The listing builds one solid part. Answer for the finished solid, in the listing's coordinates (mm). A direction names the side the tool comes from. Round coordinates to 2 decimals unless told otherwise and drop trailing zeros. Loops run counter-clockwise (first coordinate to the right, second up) from the corner with the lowest first, then second, coordinate; pieces in that order, holes last. Notation, with made-up numbers: (-14.5, 2) - (-6.5, 2) arc R19 cw to (-6.5, 35) - close; hole circle Ø1 at (11.25, -14). An arc over 180 degrees is marked (long way). One line per item, written item: value.
```python
from build123d import *

# Parameters (mm, degrees)
ESBO_O1_R                = 1.5
ESBO_O1_R_2              = 3.5
ESBO_O1_R_3              = 0.9
ESBO_O1_W                = 22.6
ESBO_O1_H                = 12.3
ESBO_O1_W_2              = 3
ESBO_O1_H_2              = 8
ESBO_O1_W_3              = 8
ESBO_O1_H_3              = 3
RESSALTO_EXTRUS_O1_DEPTH = 3


with BuildPart() as part:
    # Esboço1 → Ressalto-extrusão1 (new body)
    with BuildSketch(Plane(origin=(0, 0, 0), x_dir=(1, 0, 0), z_dir=(0, 1, 0))):
        with BuildLine():
            ThreePointArc((-26.75078073, 16.719697214), (-30.815641586, -2.3e-07), (-26.750780519, -16.719697622))
            ThreePointArc((-26.750780519, -16.719697622), (-23.767751269, -20.202130616), (-19.544028371, -21.987058612))
            add(Edge.make_bspline(
                [(23.247280819, -14.466941833), (22.21541658, -14.85491506), (7.843575487, -20.128766531), (-8.032505645, -23.945383183), (-19.544028371, -21.987058612)],
                knots=[0.1894974, 0.1894974, 0.1894974, 0.1894974, 0.216439611, 0.561126756, 0.561126756, 0.561126756, 0.561126756], degree=3))
            ThreePointArc((23.247280819, -14.466941833), (53.114593998, -6.632399806), (83.953283265, -5.079438247))
            add(Edge.make_bspline(
                [(97.598521861, -6.15), (93.039003458, -5.676054912), (88.490590593, -5.319200994), (83.953283265, -5.079438247)],
                knots=[0, 0, 0, 0, 0.137959586, 0.137959586, 0.137959586, 0.137959586], degree=3))
            add(Edge.make_bspline(
                [(114.569723425, -4.259468977), (109.134912936, -6.157348784), (103.477845748, -6.787525792), (97.598521861, -6.15)],
                knots=[0.35388944, 0.35388944, 0.35388944, 0.35388944, 1, 1, 1, 1], degree=3))
            ThreePointArc((114.569723425, -4.259468977), (117.037611185, -3.468795912), (119.543150354, -2.807050219))
            add(Edge.make_bspline(
                [(119.543150354, -2.807050219), (131.408766059, 0), (119.543150354, 2.807050219)],
                knots=[5.194112445, 5.194112445, 5.194112445, 7.372258169, 7.372258169, 7.372258169], degree=2, weights=[1, 0.463307193, 1]))
            ThreePointArc((119.543150354, 2.807050219), (117.037611185, 3.468795912), (114.569723425, 4.259468977))
            add(Edge.make_bspline(
                [(114.569723425, 4.259468977), (109.134912936, 6.157348784), (103.477845748, 6.787525792), (97.598521861, 6.15)],
                knots=[0.35388944, 0.35388944, 0.35388944, 0.35388944, 1, 1, 1, 1], degree=3))
            add(Edge.make_bspline(
                [(97.598521861, 6.15), (93.039003574, 5.676054924), (88.490590825, 5.319201013), (83.953283612, 5.079438265)],
                knots=[0, 0, 0, 0, 0.137959582, 0.137959582, 0.137959582, 0.137959582], degree=3))
            ThreePointArc((83.953283612, 5.079438265), (53.114594943, 6.632399691), (23.24728229, 14.466941345))
            add(Edge.make_bspline(
                [(23.24728229, 14.466941345), (22.21541757, 14.854914742), (7.843576153, 20.128766099), (-8.032505406, 23.945382333), (-19.544028008, 21.987058404)],
                knots=[0.189497388, 0.189497388, 0.189497388, 0.189497388, 0.216439611, 0.561126752, 0.561126752, 0.561126752, 0.561126752], degree=3))
            ThreePointArc((-19.544028008, 21.987058404), (-23.767751262, 20.202130438), (-26.75078073, 16.719697214))
        make_face()
        with Locations((-14.3, 0)):
            Circle(ESBO_O1_R, mode=Mode.SUBTRACT)
        with Locations((14.3, 0)):
            Circle(ESBO_O1_R, mode=Mode.SUBTRACT)
        with Locations((0.2, 14.3)):
            Circle(ESBO_O1_R, mode=Mode.SUBTRACT)
        with Locations((-22.8, -14.3)):
            Circle(ESBO_O1_R, mode=Mode.SUBTRACT)
        with Locations((-14.3, 11.5)):
            Circle(ESBO_O1_R, mode=Mode.SUBTRACT)
        with Locations((14.3, -11.5)):
            Circle(ESBO_O1_R, mode=Mode.SUBTRACT)
        with Locations((106.3, 0)):
            Circle(ESBO_O1_R_2, mode=Mode.SUBTRACT)
        with Locations((96.3, 0)):
            Circle(ESBO_O1_R_3, mode=Mode.SUBTRACT)
        with Locations((116.3, 0)):
            Circle(ESBO_O1_R_3, mode=Mode.SUBTRACT)
        with Locations((31.3, 0)):
            Circle(ESBO_O1_R, mode=Mode.SUBTRACT)
        with Locations((81.3, 0)):
            Circle(ESBO_O1_R, mode=Mode.SUBTRACT)
        Rectangle(ESBO_O1_W, ESBO_O1_H, mode=Mode.SUBTRACT)
        with Locations((0.2, -14.3)):
            Rectangle(ESBO_O1_W_2, ESBO_O1_H_2, mode=Mode.SUBTRACT)
        with Locations((-22.8, 14.3)):
            Rectangle(ESBO_O1_W_2, ESBO_O1_H_2, mode=Mode.SUBTRACT)
        with Locations((14.3, 11.500000009)):
            Rectangle(ESBO_O1_W_3, ESBO_O1_H_3, mode=Mode.SUBTRACT)
        with Locations((-14.3, -11.5)):
            Rectangle(ESBO_O1_W_3, ESBO_O1_H_3, mode=Mode.SUBTRACT)
        Polygon((56.3, -1.5), (60.3, -1.5), (60.3, 1.5), (52.3, 1.5), (52.3, -1.5), align=None, mode=Mode.SUBTRACT)
    extrude(amount=RESSALTO_EXTRUS_O1_DEPTH)


solid = part.part
```
1) For faces 1 (the cylindrical face through (117, 1.48, 3.48)), 2 (the flat face through (-14, 1, 10)), determine the directions among +Z, -Z, +X, -X, +Y, -Y from which every point of the face is accessible in a straight line to the end or side of a thin tool.
Final values:
face 1: +Z, +X, +Y, -Y
face 2: +Y, -Y
2) A cutting plane is placed at D-D on x = 71. Give the vertices of the cut face in (y, z).
Final values:
outline: (0, -4.96) - (3, -4.96) - (3, 4.96) - (0, 4.96) - close
3) Consider L1, parallel to Z at x = -22.5, y = 1.75; L2, parallel to Z at x = 4.5, y = 1.2; L3, parallel to Z at x = -2, y = 1.1. Determine where each line is inside the solid, lowest interval first.
Final values:
L1: -20.99 to -18.3, -10.3 to 12.83, 15.77 to 20.99
L2: -20.3 to -6.15, 6.15 to 20.3
L3: -21.6 to -6.15, 6.15 to 21.6
4) A cutting plane is placed at A-A on x = -22.8. Give the vertices of the cut face in (y, z), and give its area (3 significant figures).
Final values:
outline: (0, -20.83) - (3, -20.83) - (3, -18.3) - (0, -18.3) - close; (0, -10.3) - (3, -10.3) - (3, 12.8) - (0, 12.8) - close; (0, 15.8) - (3, 15.8) - (3, 20.83) - (0, 20.83) - close
area: 92.0 mm2
5) A cutting plane is placed at B-B on y = 1.9. Give the number of separate pieces and of enclosed holes in the cut face, and give its area (3 significant figures).
Final values:
separate pieces: 1
enclosed holes: 17
area: 2,930 mm2
6) Each of these flat-tipped pins is pushed along its axis until it touches: pin 1 Ø1.5 at (x, y) = (99.5, 2) entering from +Z; pin 2 Ø0.9 at (y, z) = (1, 12.5) entering from -X; pin 3 Ø0.9 at (x, y) = (15, 1.5) entering from +Z; pin 4 Ø4 at (x, z) = (0.2, -14.3) entering from +Y. Where does it stop, or does it pass through?
Final values:
pin 1: z = 6.35
pin 2: x = -28.76
pin 3: z = 17.5
pin 4: y = 3
7) For a pull along Z with two mould halves and no side action, classify faces 3 (the cylindrical face through (117.07, 1.48, -3.46)), 4 (the cylindrical face through (52.69, 1.48, 6.7)), 5 (the cylindrical face through (-0.125, 1.479, -12.836)) as released by +Z, released by -Z, zero draft, split by the parting line, or undercut.
Final values:
face 3: released by -Z
face 4: released by +Z
face 5: undercut
